Autodesk Inventor part; units mm, degrees
ref_plane "YZ Plane" through (0, 0, 0) normal (1, 0, 0) x (0, 1, 0)
ref_plane "XZ Plane" through (0, 0, 0) normal (0, 1, 0) x (-1, 0, 0)
ref_plane "XY Plane" through (0, 0, 0) normal (0, 0, 1) x (1, 0, 0)
sketch "Sketch1" plane through (0, 0, 0) normal (0, 1, 0) x (-1, 0, 0)
  circle A0 centre (5.98, -1.0093) radius 2.1844
  circle A1 centre (-6.72, -1.0093) radius 2.1844
  arc A2 (25.9781, -0.3931) -> (23.0279, 11.58) centre (23.0279, 5.23) ccw
  arc A3 (-24.4341, 11.9556) -> (-27.4345, -0.0172) centre (-24.4843, 5.6058) ccw
  circle A4 centre (23.0279, 5.23) radius 2.0955
  circle A5 centre (-24.4843, 5.6058) radius 2.0955
  line L0 (23.0279, 11.58) -> (-24.4341, 11.9556)
  circle A6 centre (-0.37, -20.0593) radius 2.1844
  arc A7 (-3.6903, -23.4735) -> (2.973, -23.4513) centre (-0.37, -20.0593) ccw
  line L1 (27.4853, 0.7073) -> (2.973, -23.4513)
  line L2 (-28.9114, 1.0535) -> (-3.6903, -23.4735)
  point P0 (0, 0)
  dimension "d0" = 12.7
  dimension "d1" = 12.7
  dimension "d2" = 4.191
  dimension "d3" = 4.191
  dimension "d4" = 9.525
  dimension "d7" = 6.2393
  dimension "d8" = 17.0479
extrude "Extrusion1" add sketch "Sketch1" along normal blind 1.5875
equation "\"BendRadius\" = Thickness"
equation "\"BendReliefWidth\" = Thickness"
equation "\"BendReliefDepth\" = 0.5 * Thickness"
equation "\"CornerReliefSize\" = 4 * Thickness"
equation "\"MinimumRemnant\" = 2 * Thickness"
equation "\"TransitionRadius\" = BendRadius"
equation "\"JacobiRadiusSize\" = BendRadius"
equation "\"GapSize\" = Thickness"
properties part number "MOGO Clamp Gusset" material "Acetal Resin, White"
Model file for the job. Use its own axes, mm. Round coordinates to 2 decimals unless told otherwise and drop trailing zeros. Order: outer loops, then holes, each group sorted by start corner. A loop starts at its lowest first (then second) coordinate and runs counter-clockwise, first axis right, second up. Notation, with made-up numbers: (1.25, 44.5) -> (54.25, 44.5) arc R25 ccw to (54.25, 77.5) -> close; hole circle Ø6 at (-12, 69.5). An arc over 180 degrees is marked (long way). Use one line per item in the form item = value.
Item 1: Pull direction Z, two halves, no side cores. Call faces 1 (the face through (-21.483, 0.783, 3.814)), 2 (the face through (-7.998, 0.783, -0.173)), 3 (the face through (0.3, 0.78, -24.82)), 4 (the face through (1, 1.588, -2)): released by +Z, released by -Z, zero draft, split by the parting line, or undercut.
Returned:
face_1 = undercut
face_2 = undercut
face_3 = released by -Z
face_4 = zero draft
Item 2: Cut at A-A, the plane z = -21. Write the cut outline in (x, y), and give its area (3 significant figures).
Returned:
outline = (-5.46, 0) -> (-1.6, 0) -> (-1.6, 1.59) -> (-5.46, 1.59) -> close; (2.34, 0) -> (6.23, 0) -> (6.23, 1.59) -> (2.34, 1.59) -> close
area = 12.3 mm^2
Item 3: Cut at D-D, the plane x = -15. Write the cut outline in (y, z), and give its area (3 significant figures).
Returned:
outline = (0, -11.6) -> (1.59, -11.6) -> (1.59, 11.64) -> (0, 11.64) -> close
area = 36.9 mm^2
Item 4: Drill centre lines: line 1 (X direction, y = 1.45, z = -3); line 2 (Z direction, x = -5.98, y = 0.85); line 3 (Z direction, x = 0.37, y = 1.3). Where is each one in solid material? Low to high.
Returned:
line_1 = -23.72 to -6.88, -5.08 to 5.82, 7.62 to 24.74
line_2 = -20.49 to -3.19, 1.18 to 11.71
line_3 = -24.82 to -22.24, -17.87 to 11.77
Item 5: Cut at C-C, the plane y = 0.85. Write the cut outline in (x, z) (1 decimal).
Returned:
outline = (-27.5, 0.7) -> (-3, -23.5) arc R4.8 ccw to (3.7, -23.5) -> (28.9, 1.1) arc R6.3 ccw to (24.4, 12) -> (-23, 11.6) arc R6.4 ccw to start; hole circle Ø4.2 at (-23, 5.2); hole circle Ø4.4 at (-6, -1); hole circle Ø4.4 at (0.4, -20.1); hole circle Ø4.4 at (6.7, -1); hole circle Ø4.2 at (24.5, 5.6)
Item 6: Flat gauge pin, fed straight in: pin 1 Ø5 at (x, z) = (-5.98, -1.01) entering from -Y. Where does the tip first touch, or does it go through?
Returned:
pin_1 = 0
Item 7: Cut at B-B, the plane x = 0.37. Write the cut outline in (y, z), and give its area (3 significant figures).
Returned:
outline = (0, -24.82) -> (1.59, -24.82) -> (1.59, -22.24) -> (0, -22.24) -> close; (0, -17.87) -> (1.59, -17.87) -> (1.59, 11.77) -> (0, 11.77) -> close
area = 51.1 mm^2
